Model file for the job. Use its own axes, mm. Face numbers are marked on the shaded views. A direction names the side the tool comes from. Give positions to 0.01 mm unless a question says otherwise; leave off trailing zeros. Order: outer loops, then holes, each group sorted by start corner. A loop starts at its lowest first (then second) coordinate and runs counter-clockwise, first axis right, second up. Notation, with made-up numbers: M -26.75,37 L -13.75,37 A33 ccw -13.75,73 Z; hole C -17,88 d7. An arc over 180 degrees is marked long. Return JSON: item names as keys, results as strings. Group by question number.
1. Slice it at D-D on x = 6.5. List the corners of the cut face in (y, z), then the cut area to 3 significant figures.
2. Slice it at B-B on z = 2. List the corners of the cut face in (x, y), then the cut area to 3 significant figures.
3. Two-plate mould, pull along Y, no slides. Class the marked faces 1, 2, 3 and 4: released by +Y, released by -Y, zero draft, split by the parting line, or undercut.
4. Wall check: probe 1 along Y at (x, z) = (0, 5.5); probe 2 along Z at (x, y) = (-4, -11); probe 3 along X at (y, z) = (11.5, 2). Give the ranges that are in metal, low to high. Write a range as [from, to].
5. Pin check, flat tips, straight feed: pin 1 (5 mm diameter, centred on y = -3.5, z = 4.5, fed in from +X); pin 2 (1.8 mm diameter, centred on x = 0, y = 0, fed in from -Z). Stop position of each tip, or through.
6. Slice it at C-C on y = 7. List the corners of the cut face in (x, z), then the cut area to 3 significant figures.
7. Slice it at A-A on y = 0. List the corners of the cut face in (x, z).
8. 3-axis set-ups, long thin cutter, end or side, ignore diameter. For the marked faces 5 and 6: which of +Z, -Z, +X, -X, +Y, -Y reach the whole face in a straight line?
from build123d import *

# Parameters (mm, degrees)
F0_R     = 14.5
F0_R_2   = 8.4
F1_DEPTH = 3
F2_DEPTH = 9
F3_START = 2.5
F0_R_3   = 1.5
F3_DEPTH = 6.5


with BuildPart() as f1:
    # F0 (on Top) → F1 (new body)
    with BuildSketch(Plane.XY):
        Circle(F0_R)
        Circle(F0_R_2, mode=Mode.SUBTRACT)
    extrude(amount=F1_DEPTH)

    # F0 (on Top) → F2 (join)
    with BuildSketch(Plane.XY):
        Circle(F0_R_2)
        Polygon((-2.75, -1.5877132403), (-2.75, 1.5877132403), (0, 3.1754264805), (2.75, 1.5877132403), (2.75, -1.5877132403), (0, -3.1754264805), align=None, mode=Mode.SUBTRACT)
    extrude(amount=F2_DEPTH)

    # F0 (on Top) → F3 (join)
    with BuildSketch(Plane.XY.offset(F3_START)):
        Polygon((0, 3.1754264805), (-2.75, 1.5877132403), (-2.75, -1.5877132403), (0, -3.1754264805), (2.75, -1.5877132403), (2.75, 1.5877132403), align=None)
        Circle(F0_R_3, mode=Mode.SUBTRACT)
    extrude(amount=F3_DEPTH)


solid = f1.part
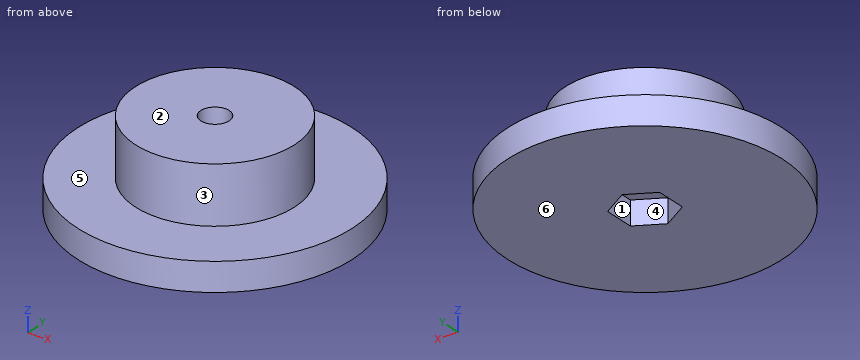
Result:
{
 "1": {"outline": "M -12.96,0 L 12.96,0 L 12.96,3 L 5.32,3 L 5.32,9 L -5.32,9 L -5.32,3 L -12.96,3 Z", "area": "142 mm2"},
 "2": {"outline": "C 0,0 d29; hole M -2.75,-1.59 L 0,-3.18 L 2.75,-1.59 L 2.75,1.59 L 0,3.18 L -2.75,1.59 Z", "area": "634 mm2"},
 "3": {"face 1": "undercut", "face 2": "zero draft", "face 3": "split by the parting line", "face 4": "undercut"},
 "4": {"probe 1": "y = [-8.4, -1.5], [1.5, 8.4]", "probe 2": "z = [0, 3]", "probe 3": "x = [-8.83, 8.83]"},
 "5": {"pin 1": "stops at x = 14.42", "pin 2": "passes through"},
 "6": {"outline": "M -12.7,0 L 12.7,0 L 12.7,3 L 4.64,3 L 4.64,9 L -4.64,9 L -4.64,3 L -12.7,3 Z", "area": "132 mm2"},
 "7": {"outline": "M -14.5,0 L -2.75,0 L -2.75,2.5 L -1.5,2.5 L -1.5,9 L -8.4,9 L -8.4,3 L -14.5,3 Z; M 1.5,2.5 L 2.75,2.5 L 2.75,0 L 14.5,0 L 14.5,3 L 8.4,3 L 8.4,9 L 1.5,9 Z"},
 "8": {"face 5": "+Z", "face 6": "-Z, +X, -X, +Y, -Y"}
}
